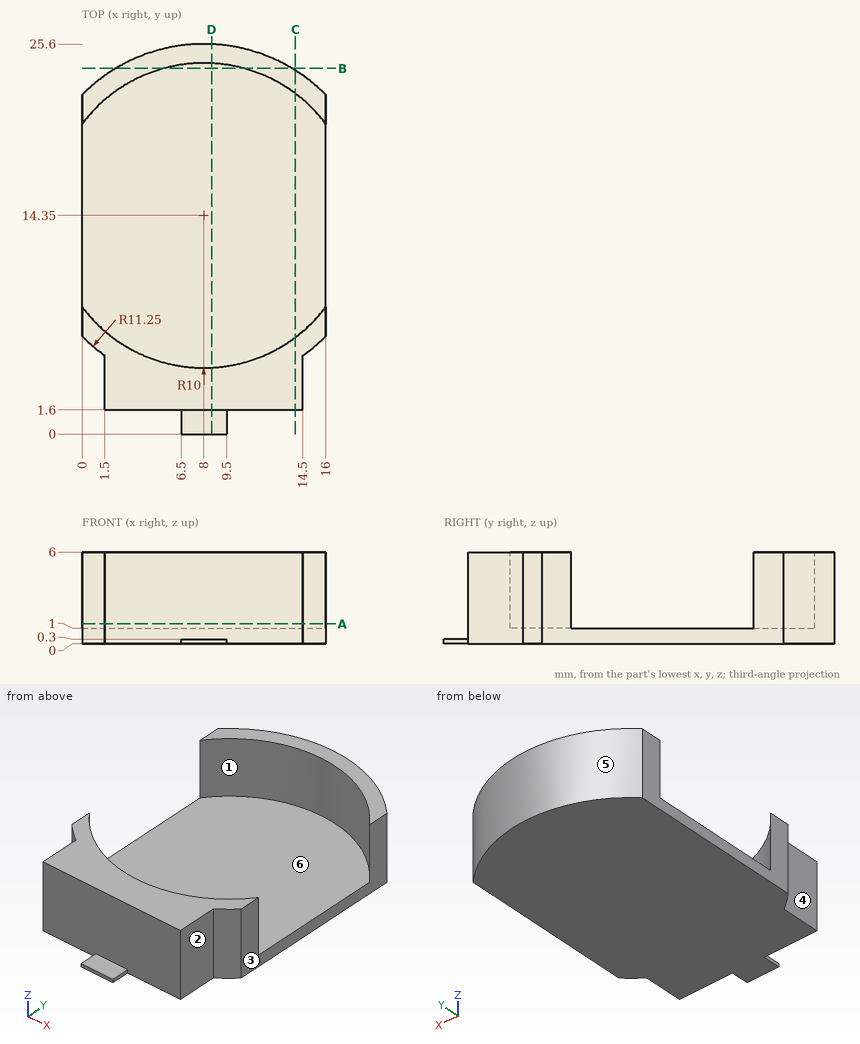
Can you work these out from the drawing? Everything is in mm from the part's minimum corner. A direction names the side the tool comes from. Round coordinates to 2 decimals unless told otherwise and drop trailing zeros. Loops run counter-clockwise (first coordinate to the right, second up) from the corner with the lowest first, then second, coordinate; pieces in that order, holes last. Notation, with made-up numbers: (-10.75, -30.5) -> (27.25, -30.5) arc R11 cw to (27.25, -11.5) -> close; hole circle Ø5 at (89, -17). An arc over 180 degrees is marked (long way). Answer in a Markdown table with one row per item.
Item 1: Suppose I cut it at D-D, the plane x = 8.5. List the corners of the cut face in (y, z) for me, plus the area to 3 significant figures.
Answer block:
| item | result |
|---|---|
| outline | (0, 0) -> (25.59, 0) -> (25.59, 6) -> (24.34, 6) -> (24.34, 1) -> (4.36, 1) -> (4.36, 6) -> (1.6, 6) -> (1.6, 0.3) -> (0, 0.3) -> close |
| area | 44.5 mm² |
Item 2: Suppose I cut it at B-B, the plane y = 24. List the corners of the cut face in (x, z) for me, plus the area to 3 significant figures.
Answer block:
| item | result |
|---|---|
| outline | (2.22, 0) -> (13.78, 0) -> (13.78, 6) -> (10.62, 6) -> (10.62, 1) -> (5.38, 1) -> (5.38, 6) -> (2.22, 6) -> close |
| area | 43.2 mm² |
Item 3: On a 3-axis mill with a long thin cutter (end or side, diameter ignored), from which of +Z, -Z, +X, -X, +Y, -Y can I reach the whole of each face in a straight line? I mean the marked faces 1, 2 and 3. Say none if no direction works.
Answer block:
| item | result |
|---|---|
| face 1 | +Z |
| face 2 | +Z, -Z, +X, -Y |
| face 3 | +Z, -Z, +X, +Y, -Y |
Item 4: Will these pins go through, and if not, where does the flat tip stop? P1, Ø1.5, axis at x = 13, z = 2.5, coming from the -Y side; P2, Ø1.8, axis at y = 2.5, z = 3.5, coming from the -X side; P3, Ø0.5, axis at x = 7.5, y = 1, coming from the +Z side.
Answer block:
| item | result |
|---|---|
| P1 | y = 1.6 |
| P2 | x = 1.5 |
| P3 | z = 0.3 |
Item 5: We'd pull the mould along Y, two halves only. Please class the marked faces 4, 5 and 6: released by +Y, released by -Y, zero draft, split by the parting line, or undercut.
Answer block:
| item | result |
|---|---|
| face 4 | zero draft |
| face 5 | released by +Y |
| face 6 | undercut |
Item 6: If I drill on probe 1 along Z at (x, y) = (11.25, 14.5); probe 2 along X at (y, z) = (21.75, 3.5); probe 3 along Y at (x, z) = (4, 2.55), over which ranges is the centre line in solid material (lowest first)?
Answer block:
| item | result |
|---|---|
| probe 1 | 0 to 1 |
| probe 2 | 0 to 1.27, 14.73 to 16 |
| probe 3 | 1.6 to 5.18, 23.52 to 24.86 |
Item 7: Suppose I cut it at C-C, the plane x = 14. List the corners of the cut face in (y, z) for me.
Answer block:
| item | result |
|---|---|
| outline | (1.6, 0) -> (23.87, 0) -> (23.87, 6) -> (22.35, 6) -> (22.35, 1) -> (6.35, 1) -> (6.35, 6) -> (1.6, 6) -> close |
Item 8: Suppose I cut it at A-A, the plane z = 1.3. List the corners of the cut face in (x, y) for me.
Answer block:
| item | result |
|---|---|
| outline | (0, 6.44) arc R11.25 ccw to (1.5, 5.17) -> (1.5, 1.6) -> (14.5, 1.6) -> (14.5, 5.17) arc R11.25 ccw to (16, 6.44) -> (16, 8.35) arc R10 cw to (0, 8.35) -> close; (0, 20.35) arc R10 cw to (16, 20.35) -> (16, 22.26) arc R11.25 ccw to (0, 22.26) -> close |
